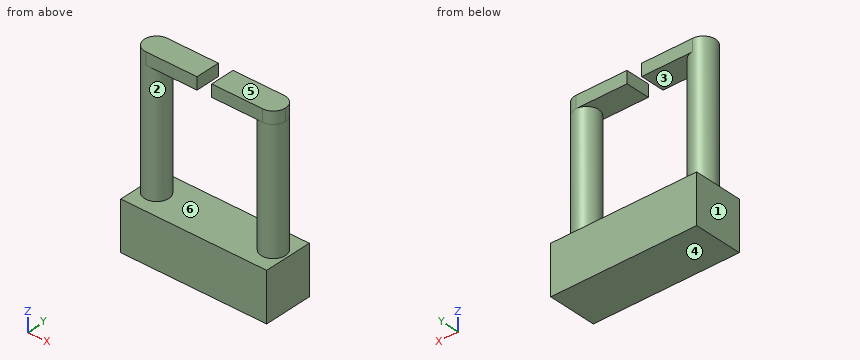
from build123d import *

# Parameters (mm, degrees)
F0_W     = 300
F0_H     = 100
F1_DEPTH = 100
F3_R     = 25
F4_DEPTH = 250
F6_DEPTH = 25
F7_DEPTH = 25
F8_W     = 30.181502
F8_H     = 25
F9_DEPTH = 75.001


with BuildPart() as f1:
    # F0 (on Top) → F1 (new body)
    with BuildSketch(Plane.XY):
        Rectangle(F0_W, F0_H)
    extrude(amount=F1_DEPTH)

    # F3 (on face) → F4 (join)
    with BuildSketch(Plane.XY.offset(100)):
        with Locations((120, 0)):
            Circle(F3_R)
        with Locations((-120, 0)):
            Circle(F3_R)
    extrude(amount=F4_DEPTH)

    # F5 (on face) → F6 (join)
    with BuildSketch(Plane.XY.offset(350)):
        with BuildLine():
            Line((120.000002, 25), (-120, 25))
            ThreePointArc((-120, 25), (-102.32233, 17.67767), (-95, 0))
            ThreePointArc((-95, 0), (-102.32233, -17.67767), (-120, -25))
            Line((-120, -25), (120.000002, -25))
            Line((120.000002, -25), (120.000002, 25))
        make_face()
        with BuildLine():
            ThreePointArc((-95, 0), (-102.32233, 17.67767), (-120, 25))
            Line((-120, 25), (-120, -25))
            ThreePointArc((-120, -25), (-102.32233, -17.67767), (-95, 0))
        make_face()
    extrude(amount=F6_DEPTH)

    # F4_face (on face) → F7 (join, through all)
    with BuildSketch(Plane(origin=(-120, 0, 350), x_dir=(1, 0, 0), z_dir=(0, 0, 1))):
        with BuildLine():
            Line((0, -25), (0, 25))
            ThreePointArc((0, 25), (-25, 0), (0, -25))
        make_face()
        with BuildLine():
            ThreePointArc((240.000002, -25), (257.67767, -17.677669), (265, 0))
            ThreePointArc((265, 0), (257.67767, 17.677669), (240.000002, 25))
            Line((240.000002, 25), (240.000002, -25))
        make_face()
    extrude(amount=F7_DEPTH)

    # F8 (on face) → F9 (cut, through all)
    with BuildSketch(Plane.XZ.offset(25)):
        with Locations((0, 362.5)):
            Rectangle(F8_W, F8_H)
    extrude(amount=-F9_DEPTH, mode=Mode.SUBTRACT)


solid = f1.part
Build history of the part. All positions in model axes, mm. Face numbers are marked on the shaded views. A direction names the side the tool comes from. Round coordinates to 2 decimals unless told otherwise and drop trailing zeros. Write each loop counter-clockwise with the first axis right and the second up, starting at its lowest first coordinate (ties: lowest second). Pieces come first, ordered by that corner, then holes. Notation, with made-up numbers: (67.5, 50) -> (93.5, 50) arc R13 cw to (93.5, 57) -> close; hole circle Ø3 at (0, 29). An arc over 180 degrees is marked (long way). Use one line per item in the form item = value.
Q1. Band-saw the part on C-C, the plane z = 316.5. Write the cut outline in (x, y).
Conclusion:
outline = circle Ø50 at (-120, 0); circle Ø50 at (120, 0)
Q2. Drill centre lines: L1, parallel to Z at x = -21, y = 19; L2, parallel to Z at x = -14, y = -15.5; L3, parallel to X at y = 3.5, z = 327.5. Where is each one in solid material? Low to high.
Conclusion:
L1 = 0 to 100, 350 to 375
L2 = 0 to 100
L3 = -144.75 to -95.25, 95.25 to 144.75
Q3. Band-saw the part on D-D, the plane x = 102. Write the cut outline in (y, z).
Conclusion:
outline = (-50, 0) -> (50, 0) -> (50, 100) -> (17.35, 100) -> (17.35, 350) -> (25, 350) -> (25, 375) -> (-25, 375) -> (-25, 350) -> (-17.35, 350) -> (-17.35, 100) -> (-50, 100) -> close
Q4. Tool access for the marked faces 5 and 6: list every direction of +Z, -Z, +X, -X, +Y, -Y with a clear straight run to the whole face (end or side of a thin tool).
Conclusion:
face_5 = +Z, +X, -X, +Y, -Y
face_6 = none
Q5. Band-saw the part on A-A, the plane x = -36. Write the cut outline in (y, z), then the cut area to 4 significant figures.
Conclusion:
outline = (-50, 0) -> (50, 0) -> (50, 100) -> (-50, 100) -> close; (-25, 350) -> (25, 350) -> (25, 375) -> (-25, 375) -> close
area = 11,250 mm²
Q6. Two-plate mould, pull along Z, no slides. Class the marked faces 1, 2, 3 and 4: released by +Z, released by -Z, zero draft, split by the parting line, or undercut.
Conclusion:
face_1 = zero draft
face_2 = undercut
face_3 = undercut
face_4 = released by -Z
Q7. Band-saw the part on B-B, the plane y = 7. Write the cut outline in (x, z), then the cut area to 3 significant figures.
Conclusion:
outline = (-150, 0) -> (150, 0) -> (150, 100) -> (144, 100) -> (144, 375) -> (15.09, 375) -> (15.09, 350) -> (96, 350) -> (96, 100) -> (-96, 100) -> (-96, 350) -> (-15.09, 350) -> (-15.09, 375) -> (-144, 375) -> (-144, 100) -> (-150, 100) -> close
area = 60,400 mm²
Q8. Drop flat-ended pins along their axis: P1, Ø12.5, axis at x = 82.5, z = 357.5, coming from the -Y side; P2, Ø4, axis at x = 108, z = 230.5, coming from the +Y side; P3, Ø1, axis at y = 0, z = 149.5, coming from the -X side; P4, Ø1, axis at y = 27, z = 127.5, coming from the +X side. Give the stop position or say it passes through.
Conclusion:
P1 = -25
P2 = 22.91
P3 = -145
P4 = through
